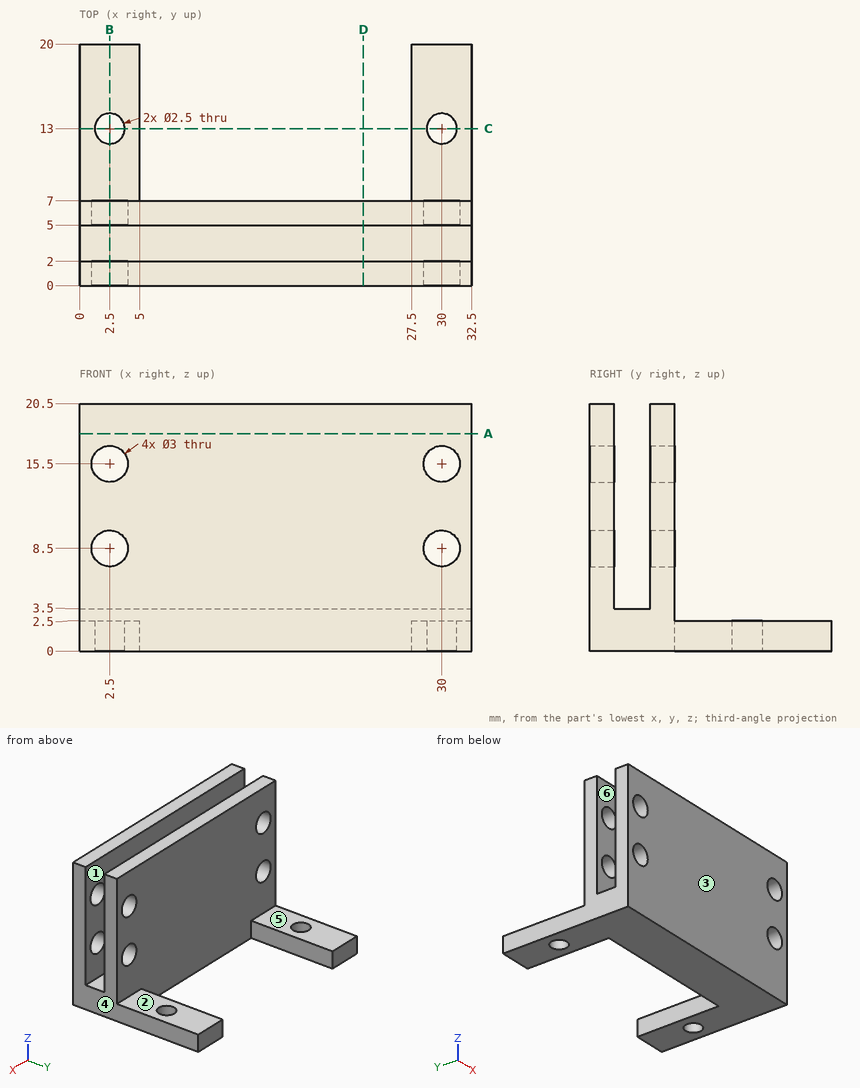
Answer from the drawing. Dimensions are ordinates in mm from the lowest x, y and z of the part. A direction names the side the tool comes from. Give positions to 0.01 mm unless a question says otherwise; leave off trailing zeros. Loops run counter-clockwise (first coordinate to the right, second up) from the corner with the lowest first, then second, coordinate; pieces in that order, holes last. Notation, with made-up numbers: (-23.75, -9.75) -> (12.25, -9.75) arc R31 cw to (12.25, 24.25) -> close; hole circle Ø2 at (23, -34.75). An arc over 180 degrees is marked (long way). Use a Markdown table: item, result.
Q1. Section A-A, the plane z = 18 is taken. Determine the outline of the cut face in (x, y), then the cut area to 3 significant figures.
Solved:
| item | result |
|---|---|
| outline | (0, 0) -> (32.5, 0) -> (32.5, 2) -> (0, 2) -> close; (0, 5) -> (32.5, 5) -> (32.5, 7) -> (0, 7) -> close |
| area | 130 mm^2 |
Q2. Determine the mould class of the marked faces 1, 2 and 3 for opening direction Y: pulls with the +Y half, pulls with the -Y half, needs draft (parallel to the pull), parting line crosses it, or undercut.
Solved:
| item | result |
|---|---|
| face 1 | undercut |
| face 2 | needs draft |
| face 3 | pulls with the -Y half |
Q3. Section C-C, the plane y = 13 is taken. Determine the outline of the cut face in (x, z), then the cut area to 3 significant figures.
Solved:
| item | result |
|---|---|
| outline | (0, 0) -> (1.25, 0) -> (1.25, 2.5) -> (0, 2.5) -> close; (3.75, 0) -> (5, 0) -> (5, 2.5) -> (3.75, 2.5) -> close; (27.5, 0) -> (28.75, 0) -> (28.75, 2.5) -> (27.5, 2.5) -> close; (31.25, 0) -> (32.5, 0) -> (32.5, 2.5) -> (31.25, 2.5) -> close |
| area | 12.5 mm^2 |
Q4. Find the intervals of material crossed by line 1 along Z through (x, y) = (2.5, 0.6); line 2 along X through (y, z) = (1.45, 8.5); line 3 along Y through (x, z) = (15.5, 12), in increasing order.
Solved:
| item | result |
|---|---|
| line 1 | z = 0 to 7, 10 to 14, 17 to 20.5 |
| line 2 | x = 0 to 1, 4 to 28.5, 31.5 to 32.5 |
| line 3 | y = 0 to 2, 5 to 7 |
Q5. A tool of negligible diameter and unlimited length cuts with its end or side. For the marked faces 4, 5 and 6, from which of +Z, -Z, +X, -X, +Y, -Y can it reach the whole face along a straight path? Write none if from no direction.
Solved:
| item | result |
|---|---|
| face 4 | +Z, -Z, +X, +Y, -Y |
| face 5 | +Z, +X, -X, +Y |
| face 6 | +Z, +X, -X |
Q6. Each of these flat-tipped pins is pushed along its axis until it touches: pin 1 (1.5 mm diameter, centred on x = 3, y = 10.5, fed in from +Z); pin 2 (6 mm diameter, centred on x = 14, z = 13.5, fed in from +Y); pin 3 (1.8 mm diameter, centred on x = 2.5, z = 8.5, fed in from +Y); pin 4 (4 mm diameter, centred on x = 23, y = 6.5, fed in from -Z). Where does it stop, or does it pass through?
Solved:
| item | result |
|---|---|
| pin 1 | stops at z = 2.5 |
| pin 2 | stops at y = 7 |
| pin 3 | passes through |
| pin 4 | stops at z = 0 |
Q7. Section B-B, the plane x = 2.5 is taken. Count the separate pieces of the cut face and the enclosed holes in it, then the cut area to 4 significant figures.
Solved:
| item | result |
|---|---|
| separate pieces | 6 |
| enclosed holes | 0 |
| area | 94.75 mm^2 |
Q8. Section D-D, the plane x = 23.5 is taken. Determine the outline of the cut face in (y, z).
Solved:
| item | result |
|---|---|
| outline | (0, 0) -> (7, 0) -> (7, 20.5) -> (5, 20.5) -> (5, 3.5) -> (2, 3.5) -> (2, 20.5) -> (0, 20.5) -> close |
